Part model, mm, in its own coordinate system. Round coordinates to 2 decimals unless told otherwise and drop trailing zeros. Loops run counter-clockwise (first coordinate to the right, second up) from the corner with the lowest first, then second, coordinate; pieces in that order, holes last.
(1) Cut at C-C on z = 1.85. Count the separate pieces of the cut face and the enclosed holes in it, then the cut area to 3 significant figures.
(2) Probe probe 1 along Y at (x, z) = (-19.05, 1.05); probe 2 along Y at (x, z) = (11, 1); probe 3 along Y at (x, z) = (-6, 2.8). List the from-to ranges inside material, lowest first.
(3) Mould opens along Y. For faces 1 (the face through (0, 9, 3.175)), 2 (the face through (0, -20, 2)), 3 (the face through (-18.638, -11.796, 1.61)) say: +Y half, -Y half, draft (parallel to the pull), parting line (faces both ways), or undercut.
(4) Cut at D-D on y = 1. List the corners of the cut face in (x, z) (3 decimals), then the cut area to 3 significant figures.
(5) Cut at A-A on x = 11. List the corners of the cut face in (y, z) (3 decimals).
(6) Flat gauge pin, fed straight in: pin 1 (3 mm diameter, centred on x = 5.5, y = 9.53, fed in from +Z). Where does the tip first touch, or does it go through?
(7) Cut at B-B on y = 10.5. List the corners of the cut face in (x, z) (3 decimals), then the cut area to 3 significant figures.
from build123d import *

# Parameters (mm, degrees)
SKETCH1_W           = 50.8
SKETCH1_H           = 40
SKETCH1_R           = 8
BOSS_EXTRUDE1_DEPTH = 3.175
FILLET1_R           = 6.35
SKETCH9_R           = 1.75
M3_THROUGH_DEPTH    = 33.484467442
SKETCH10_R          = 1.89865
CUT_EXTRUDE2_DEPTH  = 33.484467442


with BuildPart() as part:
    # Sketch1 → Boss-Extrude1 (new body)
    with BuildSketch(Plane.XY):
        Rectangle(SKETCH1_W, SKETCH1_H)
        Circle(SKETCH1_R, mode=Mode.SUBTRACT)
    extrude(amount=BOSS_EXTRUDE1_DEPTH)

    # Fillet1
    fillet1_edges = [part.edges().sort_by_distance(p)[0] for p in [
        (-25.4, 20, 1.5875),
        (25.4, 20, 1.5875),
        (25.4, -20, 1.5875),
        (-25.4, -20, 1.5875),
    ]]
    fillet(fillet1_edges, radius=FILLET1_R)

    # Sketch9 → M3-through (cut, through all)
    with BuildSketch(Plane.XY.offset(3.175)):
        with Locations((11, 0)):
            Circle(SKETCH9_R)
        with Locations((5.5, -9.526279442)):
            Circle(SKETCH9_R)
        with Locations((-5.5, -9.526279442)):
            Circle(SKETCH9_R)
        with Locations((-11, 0)):
            Circle(SKETCH9_R)
        with Locations((-5.5, 9.526279442)):
            Circle(SKETCH9_R)
        with Locations((5.5, 9.526279442)):
            Circle(SKETCH9_R)
    extrude(amount=-M3_THROUGH_DEPTH, mode=Mode.SUBTRACT)

    # Sketch10 → Cut-Extrude2 (cut, through all)
    with BuildSketch(Plane.XY.offset(3.175)):
        with Locations((19.05, -13.65)):
            Circle(SKETCH10_R)
        with Locations(Location((19.05, 13.65, 0), (0, 0, 180))):
            Circle(SKETCH10_R)
        with Locations(Location((-19.05, -13.65, 0), (0, 0, 180))):
            Circle(SKETCH10_R)
        with Locations((-19.05, 13.65)):
            Circle(SKETCH10_R)
    extrude(amount=-CUT_EXTRUDE2_DEPTH, mode=Mode.SUBTRACT)


solid = part.part
Final values:
1. separate pieces: 1
1. enclosed holes: 11
1. area: 1,690 mm2
2. probe 1: y = -20 to -15.55, -11.75 to 11.75, 15.55 to 20
2. probe 2: y = -20 to -1.75, 1.75 to 20
2. probe 3: y = -20 to -11.2, -7.85 to -5.29, 5.29 to 7.85, 11.2 to 20
3. face 1: draft
3. face 2: -Y half
3. face 3: undercut
4. outline: (-25.4, 0) - (-12.436, 0) - (-12.436, 3.175) - (-25.4, 3.175) - close; (-9.564, 0) - (-7.937, 0) - (-7.937, 3.175) - (-9.564, 3.175) - close; (7.937, 0) - (9.564, 0) - (9.564, 3.175) - (7.937, 3.175) - close; (12.436, 0) - (25.4, 0) - (25.4, 3.175) - (12.436, 3.175) - close
4. area: 92.6 mm2
5. outline: (-20, 0) - (-1.75, 0) - (-1.75, 3.175) - (-20, 3.175) - close; (1.75, 0) - (20, 0) - (20, 3.175) - (1.75, 3.175) - close
6. pin 1: passes through
7. outline: (-25.4, 0) - (-6.954, 0) - (-6.954, 3.175) - (-25.4, 3.175) - close; (-4.046, 0) - (4.046, 0) - (4.046, 3.175) - (-4.046, 3.175) - close; (6.954, 0) - (25.4, 0) - (25.4, 3.175) - (6.954, 3.175) - close
7. area: 143 mm2
